The model under review builds one solid part; all positions refer to its coordinate system, in mm. A direction names the side the tool comes from. Round coordinates to 2 decimals unless told otherwise and drop trailing zeros. Loops run counter-clockwise (first coordinate to the right, second up) from the corner with the lowest first, then second, coordinate; pieces in that order, holes last. Notation, with made-up numbers: M 22,51 L 65,51 A35 cw 65,87 Z; hole C 21.5,6 d1. An arc over 180 degrees is marked long. One line per question, with ' | ' between items.
from build123d import *

# Parameters (mm, degrees)
ESQUISSE1_W                    = 15
ESQUISSE1_H                    = 15
BOSS_EXTRU_1_DEPTH             = 15
TROUS_DE_CENTRAGE_5_0MM1_D     = 6.4
TROUS_DE_CENTRAGE_5_0MM1_DEPTH = 10
TROUS_DE_CENTRAGE_5_0MM1_TIP   = 1.922753981
BOSS_EXTRU_2_DEPTH             = 20
BOSS_EXTRU_2_DEPTH_BACK        = 10
ESQUISSE4_R                    = 20.6
ESQUISSE4_R_2                  = 18.6
ESQUISSE5_R                    = 16
BOSS_EXTRU_3_DEPTH             = 5
CONG_1_R                       = 20
CONG_2_R                       = 1
TROUS_DE_CENTRAGE_1_0MM1_D     = 1


with BuildPart() as part:
    # Esquisse1 → Boss.-Extru.1 (new body)
    with BuildSketch(Plane.XY):
        Rectangle(ESQUISSE1_W, ESQUISSE1_H)
    extrude(amount=BOSS_EXTRU_1_DEPTH)

    # Trous de centrage Ø5.0mm1
    with Locations(Plane(origin=(0, 0, 0), x_dir=(-1, 0, 0), z_dir=(0, 0, -1))):
        with Locations((0, 0)):
            Hole(TROUS_DE_CENTRAGE_5_0MM1_D / 2, depth=TROUS_DE_CENTRAGE_5_0MM1_DEPTH)
            with Locations((0, 0, -(TROUS_DE_CENTRAGE_5_0MM1_DEPTH + TROUS_DE_CENTRAGE_5_0MM1_TIP / 2))):  # 118° drill point
                Cone(0, TROUS_DE_CENTRAGE_5_0MM1_D / 2, TROUS_DE_CENTRAGE_5_0MM1_TIP, mode=Mode.SUBTRACT)

    # Esquisse4 → Boss.-Extru.2 (add, two sides: drawn at the far end of the back side and taken through both)
    with BuildSketch(Plane(origin=(0, 7.5, 0), x_dir=(1, 0, 0), z_dir=(0, 1, 0)).offset(-BOSS_EXTRU_2_DEPTH_BACK)):
        with Locations(Location((0, -34.186192952, 0), (0, 0, 270))):
            Circle(ESQUISSE4_R)
        with Locations(Location((0, -34.186192952, 0), (0, 0, 270))):
            Circle(ESQUISSE4_R_2, mode=Mode.SUBTRACT)
    extrude(amount=BOSS_EXTRU_2_DEPTH + BOSS_EXTRU_2_DEPTH_BACK)

    # Esquisse5 → Boss.-Extru.3 (add)
    with BuildSketch(Plane.XZ.offset(2.5)):
        with BuildLine():
            Line((-7.5, 15), (7.5, 15))
            ThreePointArc((7.5, 15), (0, 54.786192952), (-7.5, 15))
        make_face()
        with Locations(Location((0, 34.186192952, 0), (0, 0, 90))):
            Circle(ESQUISSE5_R, mode=Mode.SUBTRACT)
    extrude(amount=BOSS_EXTRU_3_DEPTH)

    # Congé1
    cong_1_edges = [part.edges().sort_by_distance(p)[0] for p in [
        (-7.5, 2.5, 15),
        (7.5, 2.5, 15),
    ]]
    fillet(cong_1_edges, radius=CONG_1_R)

    # Congé2
    cong_2_edges = [part.edges().sort_by_distance(p)[0] for p in [
        (-7.5, 0, 0),
        (7.5, 0, 0),
    ]]
    fillet(cong_2_edges, radius=CONG_2_R)

    # Trous de centrage Ø1.0mm1 (through all)
    with Locations(Plane(origin=(0, 7.5, 0), x_dir=(1, 0, 0), z_dir=(0, 1, 0))):
        with Locations((6, -13.54037013)):
            Hole(TROUS_DE_CENTRAGE_1_0MM1_D / 2)


solid = part.part
1) For line 1 (Y direction, x = 0, z = 6); line 2 (Z direction, x = 6, y = -1.5); line 3 (Y direction, x = 5, z = 11.5), list the stretches that pass through material, from the lowest coordinate up.
Output values:
line 1: y = -7.5 to -3.2, 3.2 to 7.5 | line 2: z = 0 to 13.04, 14.04 to 16.58, 51.79 to 53.89 | line 3: y = -7.5 to 7.5
2) Add section C-C on y = 22. State the section outline as (x, z) points.
Output values:
outline: C 0,34.19 d41.2; hole C 0,34.19 d37.2
3) Add section A-A on x = 4.5. State the section outline as (y, z) points.
Output values:
outline: M -7.5,0 L 7.5,0 L 7.5,14.08 L 27.5,14.08 L 27.5,16.14 L -2.5,16.14 L -2.5,18.83 L -7.5,18.83 Z; M -7.5,49.54 L -2.5,49.54 L -2.5,52.23 L 27.5,52.23 L 27.5,54.29 L -7.5,54.29 Z
4) Add section D-D on z = 47.5. State the section outline as (x, y) points.
Output values:
outline: M -15.72,-7.5 L -8.87,-7.5 L -8.87,-2.5 L -12.99,-2.5 L -12.99,27.5 L -15.72,27.5 Z; M 8.87,-7.5 L 15.72,-7.5 L 15.72,27.5 L 12.99,27.5 L 12.99,-2.5 L 8.87,-2.5 Z
5) Machinability: for faces 5 (the flat face through (15.4, 27.5, 23.4)), 6 (the flat face through (8.2, -2.5, 48.1)), 7 (the flat face through (-7.5, 0, 3)), 8 (the cylindrical face through (-2.539, -1.947, 5.07)), 9 (the cylindrical face through (15.62, -4.96, 30.72)), which of the approach directions +Z, -Z, +X, -X, +Y, -Y give a long, thin tool a straight path to every point of the face, cutting with its end or side? Answer none if there is none.
Output values:
face 5: +Z, -Z, +X, -X, +Y | face 6: +Y | face 7: -Z, -X, +Y, -Y | face 8: -Z | face 9: +Y, -Y
6) Mouldability with a two-part tool opening along X and no side actions: class faces 1 (the flat face through (7.5, 0, 3)), 2 (the cylindrical face through (-9.231, -0.105, 12.457)), 3 (the cylindrical face through (-11.32, 12.29, 19.43)), 4 (the flat face through (8, -7.5, 19)) as +X half, -X half, draft (parallel to the pull), parting line (faces both ways), or undercut.
Output values:
face 1: +X half | face 2: -X half | face 3: undercut | face 4: draft
7) Insertion check: P1, Ø5, axis at x = -6.5, y = -2, coming from the +Z side; P2, Ø1, axis at x = 14.5, z = 41, coming from the +Y side; P3, Ø22.5, axis at x = 0, z = 34.19, coming from the +Y side; P4, Ø9.5, axis at x = 6.5, z = 7.5, coming from the +Y side. Each pin has a flat end and moves straight along its axis. Give the tip position at first contact, or say it passes through.
Output values:
P1: stops at z = 54.39 | P2: stops at y = -2.5 | P3: passes through | P4: stops at y = 7.5
8) Add section B-B on z = 21. State the section outline as (x, y) points, then the cut area to 3 significant figures.
Output values:
outline: M -15.83,-7.5 L -9.06,-7.5 L -9.06,-2.5 L -13.12,-2.5 L -13.12,27.5 L -15.83,27.5 Z; M 9.06,-7.5 L 15.83,-7.5 L 15.83,27.5 L 13.12,27.5 L 13.12,-2.5 L 9.06,-2.5 Z | area: 230 mm²
